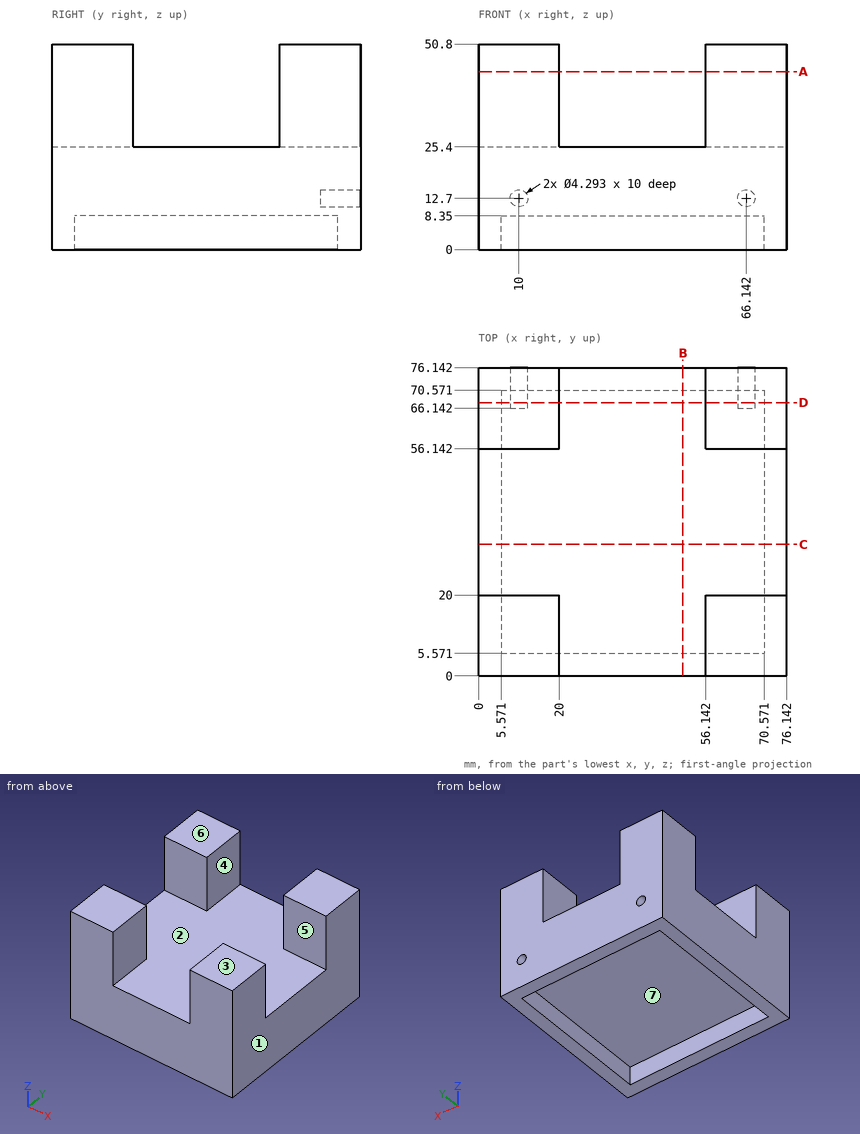
The drawing under review shows one solid part. Ordinate dimensions are in mm from its lowest x, y, z. A direction names the side the tool comes from. Coordinates: 2 decimals unless noted, no trailing zeros. Loops run counter-clockwise (first coordinate to the right, second up) from the corner with the lowest first, then second, coordinate; pieces in that order, holes last. Notation, with made-up numbers: M 71.5,76 L 94.5,76 A35 ccw 94.5,109 Z; hole C -15.75,77 d11. An arc over 180 degrees is marked long. Use one line per item in the form item = value.
(1) For the marked faces 4, 5, 6 and 7, list the 3-axis set-ups (+Z, -Z, +X, -X, +Y, -Y) from which the entire face can be reached by the end or side of a thin tool; tool diameter is ignored.
Return value:
face_4 = +Z, +Y, -Y
face_5 = +Z, +X, -X
face_6 = +Z, +X, -X, +Y, -Y
face_7 = -Z
(2) For line 1 along Y through (x, z) = (9, 36); line 2 along X through (y, z) = (62.5, 4.5); line 3 along X through (y, z) = (74, 12), list the stretches that pass through material, from the lowest coordinate up. Write a range as from..to.
Return value:
line_1 = 0..20, 56.14..76.14
line_2 = 0..5.57, 70.57..76.14
line_3 = 0..7.97, 12.03..64.11, 68.17..76.14
(3) Consider section A-A (z = 44). Write out the cut boundary in (x, y).
Return value:
outline = M 0,0 L 20,0 L 20,20 L 0,20 Z; M 0,56.14 L 20,56.14 L 20,76.14 L 0,76.14 Z; M 56.14,0 L 76.14,0 L 76.14,20 L 56.14,20 Z; M 56.14,56.14 L 76.14,56.14 L 76.14,76.14 L 56.14,76.14 Z
(4) Consider section B-B (x = 50.5). Write out the cut boundary in (y, z).
Return value:
outline = M 0,0 L 5.57,0 L 5.57,8.35 L 70.57,8.35 L 70.57,0 L 76.14,0 L 76.14,25.4 L 0,25.4 Z
(5) Draft analysis for pull direction X (two halves, no side actions). For the marked faces 1, 2 and 3, state which applies: pulls with the +X half, pulls with the -X half, needs draft (parallel to the pull), parting line crosses it, or undercut.
Return value:
face_1 = pulls with the +X half
face_2 = undercut
face_3 = needs draft
(6) Consider section D-D (y = 67.5). Write out the cut boundary in (x, z), and give its area (3 significant figures).
Return value:
outline = M 0,0 L 5.57,0 L 5.57,8.35 L 70.57,8.35 L 70.57,0 L 76.14,0 L 76.14,50.8 L 56.14,50.8 L 56.14,25.4 L 20,25.4 L 20,50.8 L 0,50.8 Z; hole C 10,12.7 d4.29; hole C 66.14,12.7 d4.29
area = 2,380 mm2
(7) Clearance check with flat-ended pins moving along their axes: P1, Ø8, axis at x = 57, y = 18, coming from the -Z side; P2, Ø3.5, axis at x = 66.14, z = 12.7, coming from the +Y side; P3, Ø6, axis at x = 27, z = 31, coming from the -Y side; P4, Ø12, axis at x = 23, y = 50, coming from the +Z side. State where each tip first meets the part, or that it passes through.
Return value:
P1 = 8.35
P2 = 66.14
P3 = through
P4 = 25.4
